Verification items for the finished model (mm, model axes). Face numbers are marked on the shaded views. A direction names the side the tool comes from. Coordinates: 2 decimals unless noted, no trailing zeros. Loops run counter-clockwise (first coordinate to the right, second up) from the corner with the lowest first, then second, coordinate; pieces in that order, holes last. Notation, with made-up numbers: M 51,46 L 55,46 A22 ccw 55,69 Z; hole C -22,-17.75 d5. An arc over 180 degrees is marked long. Write item = value, one per line. Start each with the question number.
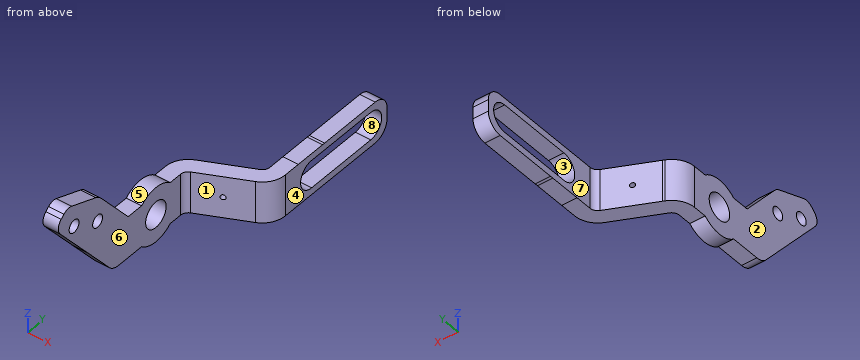
```python
from build123d import *

# Parameters (mm, degrees)
BASE_FLANGE1_START      = -3.048
BASE_FLANGE1_OUTLINE_R  = 2.6
BASE_FLANGE1_DEPTH      = 3.048
CHAMFER1_SIZE           = 5.5
CHAMFER1_SIZE2          = 9.526279442
FILLET5_R               = 3
JOG1_START              = -31.942217141
JOG1_DEPTH              = 22.299805307
JOG1_START_2            = -30.592217141
JOG1_2_DEPTH            = 1.375
JOG1_START_3            = -23.667217141
JOG1_3_DEPTH            = 1.375
JOG1_START_4            = -30.595801154
JOG1_4_DEPTH            = 8.307168025
JOG1_5_DEPTH            = 13
EDGE_FLANGE1_DEPTH      = 15
FILLET4_R               = 3
CUT_EXTRUDE4_DEPTH      = 85.269968197
CUT_EXTRUDE4_DEPTH_BACK = 85.269968197
M3X0_5_TAPPED_HOLE2_D   = 2.5
CUT_EXTRUDE5_REACH      = 59.699
SKETCH19_R              = 0.5
CUT_EXTRUDE6_DEPTH      = 80.832983383
FILLET9_R               = 2


with BuildPart() as part:
    # Base-Flange1: read off the stored shape, not the designer's step
    # Base-Flange1 outline → Base-Flange1 (new body)
    with BuildSketch(Plane(origin=(0, 0, 0), x_dir=(0, 0, -1), z_dir=(1, 0, 0)).offset(BASE_FLANGE1_START)):
        with BuildLine():
            Line((11.442217141, 3.034903463), (29.520579971, 18.204451045))
            ThreePointArc((29.520579971, 18.204451045), (30.311140503, 19.234729589), (30.592217141, 20.502584374))
            Line((30.592217141, 20.502584374), (30.592217141, 26.390637175))
            ThreePointArc((30.592217141, 26.390637175), (31.942217141, 30), (30.592217141, 33.609362825))
            Line((30.592217141, 33.609362825), (30.592217141, 49.531723164))
            Line((30.592217141, 49.531723164), (30.595801154, 55.658476217))
            Line((30.595801154, 55.658476217), (30.592217141, 56.218276836))
            Line((30.592217141, 56.218276836), (30.592217141, 72))
            Line((30.592217141, 72), (22.292217141, 72))
            Line((22.292217141, 72), (22.292217141, 56.218276836))
            Line((22.292217141, 56.218276836), (22.288633129, 55.658476217))
            Line((22.288633129, 55.658476217), (22.292217141, 49.531723164))
            Line((22.292217141, 49.531723164), (22.292217141, 33.609362825))
            ThreePointArc((22.292217141, 33.609362825), (20.942217141, 30), (22.292217141, 26.390637175))
            Line((22.292217141, 26.390637175), (22.292217141, 22.974014962))
            Line((22.292217141, 22.974014962), (6.107079981, 9.393072341))
            Line((6.107079981, 9.393072341), (11.442217141, 3.034903463))
        make_face()
        with Locations((26.442217141, 30)):
            Circle(BASE_FLANGE1_OUTLINE_R, mode=Mode.SUBTRACT)
        with BuildLine():
            ThreePointArc((23.667217141, 67.875), (26.442217141, 70.65), (29.217217141, 67.875))
            Line((29.217217141, 67.875), (29.217217141, 52.875))
            ThreePointArc((29.217217141, 52.875), (26.442217141, 50.1), (23.667217141, 52.875))
            Line((23.667217141, 52.875), (23.667217141, 67.875))
        make_face(mode=Mode.SUBTRACT)
    extrude(amount=BASE_FLANGE1_DEPTH)

    # Chamfer1
    chamfer1_edges = [part.edges().sort_by_distance(p)[0] for p in [
        (-1.524, 9.393072341, -6.107079981),
    ]]
    chamfer1_side = [part.faces().sort_by_distance(p)[0] for p in [
        (-1.524, 6.213987902, -8.774648561),
    ]]
    chamfer(chamfer1_edges, length=CHAMFER1_SIZE, length2=CHAMFER1_SIZE2, reference=chamfer1_side[0])

    # Fillet5
    fillet5_edges = [part.edges().sort_by_distance(p)[0] for p in [
        (-1.524, 15.516446733, -13.404633411),
    ]]
    fillet(fillet5_edges, radius=FILLET5_R)

    # Jog1: read off the stored shape, not the designer's step
    # Jog1 outline → Jog1 (cut)
    with BuildSketch(Plane.XY.offset(JOG1_START)):
        with BuildLine():
            Line((-0.408210693, 40.414716045), (0, 40.605067817))
            Line((0, 40.605067817), (0, 72))
            Line((0, 72), (-3.048, 72))
            Line((-3.048, 72), (-3.048, 36.271076843))
            ThreePointArc((-3.048, 36.271076843), (-2.33198569, 38.727610652), (-0.408210693, 40.414716045))
        make_face()
    extrude(amount=JOG1_DEPTH, mode=Mode.SUBTRACT)

    # Jog1 2 outline → Jog1 2 (add)
    with BuildSketch(Plane.XY.offset(JOG1_START_2)):
        with BuildLine():
            ThreePointArc((0, 36.271076843), (0.238671437, 37.089921446), (0.879929769, 37.65228991))
            Line((0.879929769, 37.65228991), (10.360210693, 42.073017507))
            ThreePointArc((10.360210693, 42.073017507), (12.28398569, 43.7601229), (13, 46.216656709))
            Line((13, 46.216656709), (13, 72))
            Line((13, 72), (9.952, 72))
            Line((9.952, 72), (9.952, 46.216656709))
            ThreePointArc((9.952, 46.216656709), (9.713328563, 45.397812106), (9.072070231, 44.835443641))
            Line((9.072070231, 44.835443641), (0, 40.605067817))
            Line((0, 40.605067817), (0, 36.271076843))
        make_face()
    extrude(amount=JOG1_2_DEPTH)

    # Jog1 3 outline → Jog1 3 (add)
    with BuildSketch(Plane.XY.offset(JOG1_START_3)):
        with BuildLine():
            ThreePointArc((0, 36.271076843), (0.238671437, 37.089921446), (0.879929769, 37.65228991))
            Line((0.879929769, 37.65228991), (10.360210693, 42.073017507))
            ThreePointArc((10.360210693, 42.073017507), (12.28398569, 43.7601229), (13, 46.216656709))
            Line((13, 46.216656709), (13, 72))
            Line((13, 72), (9.952, 72))
            Line((9.952, 72), (9.952, 46.216656709))
            ThreePointArc((9.952, 46.216656709), (9.713328563, 45.397812106), (9.072070231, 44.835443641))
            Line((9.072070231, 44.835443641), (0, 40.605067817))
            Line((0, 40.605067817), (0, 36.271076843))
        make_face()
    extrude(amount=JOG1_3_DEPTH)

    # Jog1 4 outline → Jog1 4 (add)
    with BuildSketch(Plane.XY.offset(JOG1_START_4)):
        with BuildLine():
            ThreePointArc((0, 36.271076843), (0.238671437, 37.089921446), (0.879929769, 37.65228991))
            Line((0.879929769, 37.65228991), (10.360210693, 42.073017507))
            ThreePointArc((10.360210693, 42.073017507), (12.28398569, 43.7601229), (13, 46.216656709))
            Line((13, 46.216656709), (13, 72))
            Line((13, 72), (9.952, 72))
            Line((9.952, 72), (9.952, 46.216656709))
            ThreePointArc((9.952, 46.216656709), (9.713328563, 45.397812106), (9.072070231, 44.835443641))
            Line((9.072070231, 44.835443641), (0, 40.605067817))
            Line((0, 40.605067817), (0, 36.271076843))
        make_face()
    extrude(amount=JOG1_4_DEPTH)

    # Jog1 5 outline → Jog1 5 (cut)
    with BuildSketch(Plane.YZ):
        Polygon((49.531723164, -30.592217141), (35, -30.592217141), (35, -30.595801154), (55.658476217, -30.595801154), align=None)
        Polygon((35, -22.288633129), (35, -22.292217141), (49.531723164, -22.292217141), (55.658476217, -22.288633129), align=None)
        Polygon((56.218276836, -30.592217141), (55.658476217, -30.595801154), (73, -30.595801154), (73, -30.592217141), align=None)
        Polygon((73, -22.288633129), (55.658476217, -22.288633129), (56.218276836, -22.292217141), (73, -22.292217141), align=None)
        with BuildLine():
            Line((67.875, -23.667217141), (52.875, -23.667217141))
            ThreePointArc((52.875, -23.667217141), (50.1, -26.442217141), (52.875, -29.217217141))
            Line((52.875, -29.217217141), (67.875, -29.217217141))
            ThreePointArc((67.875, -29.217217141), (70.65, -26.442217141), (67.875, -23.667217141))
        make_face()
    extrude(amount=JOG1_5_DEPTH, mode=Mode.SUBTRACT)

    # Edge-Flange1: sheet metal written as solids
    # Edge-Flange1 section (on a plane across the edge) → Edge-Flange1 (add)
    with BuildSketch(Plane(origin=(0, 1.867451731, -12.421825459), x_dir=(3.4914813388431326e-15, 0.7660444431189821, 0.6427876096865346), z_dir=(0, 0.6427876096865346, -0.7660444431189821))):
        with BuildLine():
            Line((-3.048, 1.524), (-3.048, 29.952))
            Line((-3.048, 29.952), (0, 29.952))
            Line((0, 29.952), (0, 1.524))
            ThreePointArc((0, 1.524), (0.446369265, 0.446369265), (1.524, 0))
            Line((1.524, 0), (1.524, -3.048))
            ThreePointArc((1.524, -3.048), (-1.708892204, -1.708892204), (-3.048, 1.524))
        make_face()
    extrude(amount=EDGE_FLANGE1_DEPTH)

    # Fillet4
    fillet4_edges = [part.edges().sort_by_distance(p)[0] for p in [
        (11.476, 72, -30.592217141),
        (11.476, 72, -22.292217141),
    ]]
    fillet(fillet4_edges, radius=FILLET4_R)

    # Sketch17 → Cut-Extrude4 (cut, two sides: drawn at the far end of the back side and taken through both)
    with BuildSketch(Plane(origin=(0, 0, 0), x_dir=(0, 0, -1), z_dir=(1, 0, 0)).offset(-CUT_EXTRUDE4_DEPTH_BACK)):
        Polygon((22.932883788, 12.676717608), (2.605814743, -4.379718531), (8.769545562, -11.725366877), (29.096614607, 5.331069261), align=None)
    extrude(amount=CUT_EXTRUDE4_DEPTH + CUT_EXTRUDE4_DEPTH_BACK, mode=Mode.SUBTRACT)

    # M3x0.5 Tapped Hole2 (through all)
    with Locations(Plane(origin=(-3.048, 15.221364604, -18.186856854), x_dir=(0, 0, -1), z_dir=(-1, 0, 0))):
        with Locations((0, 0), (-2.828600732, 5.963347877)):
            Hole(M3X0_5_TAPPED_HOLE2_D / 2)

    # Sketch19 → Cut-Extrude5 (cut, up to next)
    with BuildSketch(Plane(origin=(-15.552643282, 33.35275115, 0), x_dir=(0.906307787036651, 0.4226182617406973, 0), z_dir=(-0.4226182617406973, 0.906307787036651, 0)), mode=Mode.PRIVATE) as cut_extrude5_sk1:
        with Locations(Location((21.940198833, 26.442217141, 0), (0, 0, 180))):
            Circle(SKETCH19_R)
    cut_extrude5_tool1 = extrude(cut_extrude5_sk1.sketch, amount=-CUT_EXTRUDE5_REACH, mode=Mode.PRIVATE) & part.part
    add(cut_extrude5_tool1.solids().sort_by_distance((4.33193, 42.62508, -26.442217))[0], mode=Mode.SUBTRACT)

    # Sketch21 → Cut-Extrude6 (cut, through all)
    with BuildSketch(Plane(origin=(0, 0, 0), x_dir=(0, 0, -1), z_dir=(1, 0, 0))):
        Polygon((10.514234213, 7.575140201), (9.642411834, 5.179827903), (11.442217141, 3.034903463), (13.133284575, 4.453877523), align=None)
    extrude(amount=-CUT_EXTRUDE6_DEPTH, mode=Mode.SUBTRACT)

    # Fillet9
    fillet9_edges = [part.edges().sort_by_distance(p)[0] for p in [
        (-1.524, 7.575140201, -10.514234213),
        (-1.524, 4.453877523, -13.133284575),
    ]]
    fillet(fillet9_edges, radius=FILLET9_R)


solid = part.part
```
Q1. Gauge pin test, flat ends, axial feed: pin 1 (4 mm diameter, centred on y = 64.5, z = -28, fed in from -X); pin 2 (0.9 mm diameter, centred on x = -1.5, y = 25, fed in from -Z); pin 3 (1.5 mm diameter, centred on x = 12, y = 61, fed in from +Z); pin 4 (8 mm diameter, centred on x = 1.5, z = -15.5, fed in from -Y). Record the tip position at first contact, or that the pin passes through.
Q2. Sectioned sample at D-D on y = 47.5. Record the cut outline in (x, z), plus the area to 3 significant figures.
Q3. Scan lines: L1, parallel to X at y = 65.5, z = -29.25; L2, parallel to X at y = 24, z = -27; L3, parallel to Y at x = -0.25, z = -24.5. Record each from-to range of solid material in increasing order. Write a range as [from, to].
Q4. Sectioned sample at B-B on z = -18.75. Record the cut outline in (x, y).
Q5. Mould release check, pull along Y, two halves, no side actions. Record for the marked faces 1, 2 and 3: +Y half, -Y half, draft (parallel to the pull), parting line (faces both ways), or undercut.
Q6. Sectioned sample at A-A on y = 61. Record the cut outline in (x, z), plus the area to 3 significant figures.
Q7. Set-up check for the marked faces 4, 5, 6, 7 and 8: record each of +Z, -Z, +X, -X, +Y, -Y from which the full face is reachable in a straight line by a thin tool's end or side.
Q8. Sectioned sample at C-C on x = 11. Record the cut outline in (y, z) (3 decimals).
Solutions:
q1.pin_1 = 9.95
q1.pin_2 = -30.59
q1.pin_3 = -22.29
q1.pin_4 = 5.27
q2.outline = M 9.95,-30.59 L 13,-30.59 L 13,-22.29 L 9.95,-22.29 Z
q2.area = 25.3 mm²
q3.L1 = [9.95, 13]
q3.L2 = [-3.05, 0]
q3.L3 = [13.99, 28.27], [31.73, 40.49]
q4.outline = M -3.05,9.17 L 0,9.17 L 0,14.11 L -3.05,14.11 Z; M -3.05,16.34 L 0,16.34 L 0,20 L -3.05,20 Z
q5.face_1 = -Y half
q5.face_2 = draft
q5.face_3 = undercut
q6.outline = M 9.95,-30.59 L 13,-30.59 L 13,-29.22 L 9.95,-29.22 Z; M 9.95,-23.67 L 13,-23.67 L 13,-22.29 L 9.95,-22.29 Z
q6.area = 8.38 mm²
q7.face_4 = +Z, -Z, +X, +Y, -Y
q7.face_5 = +Z, +X, -X
q7.face_6 = +Z, -Z, +X, -Y
q7.face_7 = +Z, -Z, -X, +Y
q7.face_8 = +X, -X
q8.outline = M 42.437,-30.592 L 49.532,-30.592 L 55.658,-30.596 L 56.218,-30.592 L 69,-30.592 A3 ccw 72,-27.592 L 72,-25.292 A3 ccw 69,-22.292 L 56.218,-22.292 L 55.658,-22.289 L 49.532,-22.292 L 42.437,-22.292 Z; hole M 52.875,-29.217 L 67.875,-29.217 A2.775 ccw 67.875,-23.667 L 52.875,-23.667 A2.775 ccw Z
